Read the model definition and answer for the solid it produces. Units are mm, in the model's axes. A direction names the side the tool comes from. Coordinates: 2 decimals unless noted, no trailing zeros. Loops run counter-clockwise (first coordinate to the right, second up) from the corner with the lowest first, then second, coordinate; pieces in that order, holes last. Notation, with made-up numbers: M 36,-28 L 69,-28 A18 cw 69,-19 Z; hole C 5.5,-19 d3. An arc over 180 degrees is marked long. One line per item, written item: value. Start each with the question number.
1. The part is cut by section B-B (z = 3.45). Write down the section's boundary in (x, y) (3 decimals), then the cut area to 3 significant figures.
2. The part is cut by section D-D (y = 17). Write down the section's boundary in (x, z) (3 decimals).
3. The part is cut by section C-C (x = 62). Write down the section's boundary in (y, z) (3 decimals).
4. For faces 1 (the face through (39, 50.8, 3)), 2 (the face through (72.12, 46.67, 3.51)), 3 (the face through (6.979, 25, 1)), determine the directions among +Z, -Z, +X, -X, +Y, -Y from which every point of the face is accessible in a straight line to the end or side of a thin tool.
5. Determine the mould class of faces 4 (the face through (76.2, 25, 3)), 5 (the face through (39, 47.625, 4)), 6 (the face through (1.91, 48.99, 2.5)) for opening direction X: +X half, -X half, draft (parallel to the pull), parting line (faces both ways), or undercut.
6. Consider probe 1 along Y at (x, z) = (68.5, 3.4) (3 decimals); probe 2 along X at (y, z) = (34, 2) (3 decimals); probe 3 along Z at (x, y) = (41, 23.5) (3 decimals). Determine where each line is inside the solid, lowest interval first.
7. Flat-ended cylindrical pins translate along their axes: pin 1 (1.4 mm diameter, centred on x = 5, z = 1, fed in from +Y); pin 2 (0.6 mm diameter, centred on x = 5, z = 1, fed in from -Y). Find the tip coordinate at first contact, or state that the pin passes through.
8. The part is cut by section A-A (y = 24.5). Write down the section's boundary in (x, z) (3 decimals), then the cut area to 3 significant figures.
```python
from build123d import *

# Parameters (mm, degrees)
F1_DEPTH = 5.08
F3_DEPTH = 3.175
F5_DEPTH = 25.4


with BuildPart() as f1:
    # F0 (on Top) → F1 (new body)
    with BuildSketch(Plane.XY):
        with BuildLine():
            ThreePointArc((0, 6.35), (1.859872, 1.859872), (6.35, 0))
            Line((6.35, 0), (69.85, 0))
            ThreePointArc((69.85, 0), (74.340128, 1.859872), (76.2, 6.35))
            Line((76.2, 6.35), (76.2, 44.45))
            ThreePointArc((76.2, 44.45), (74.340128, 48.940128), (69.85, 50.8))
            Line((69.85, 50.8), (6.35, 50.8))
            ThreePointArc((6.35, 50.8), (1.859872, 48.940128), (0, 44.45))
            Line((0, 44.45), (0, 6.35))
        make_face()
    extrude(amount=F1_DEPTH)

    # F2 (on face) → F3 (cut)
    with BuildSketch(Plane.XY.offset(5.08)):
        with BuildLine():
            Line((69.85, 47.625), (6.35, 47.625))
            ThreePointArc((6.35, 47.625), (4.104936, 46.695064), (3.175, 44.45))
            Line((3.175, 44.45), (3.175, 6.35))
            ThreePointArc((3.175, 6.35), (4.104936, 4.104936), (6.35, 3.175))
            Line((6.35, 3.175), (69.85, 3.175))
            ThreePointArc((69.85, 3.175), (72.095064, 4.104936), (73.025, 6.35))
            Line((73.025, 6.35), (73.025, 44.45))
            ThreePointArc((73.025, 44.45), (72.095064, 46.695064), (69.85, 47.625))
        make_face()
    extrude(amount=-F3_DEPTH, mode=Mode.SUBTRACT)

    # F4 (on Top) → F5 (cut)
    with BuildSketch(Plane.XY):
        with BuildLine():
            Line((5.708611, 28.575), (4.445, 28.575))
            ThreePointArc((4.445, 28.575), (3.546974, 28.203026), (3.175, 27.305))
            Line((3.175, 27.305), (3.175, 23.495))
            ThreePointArc((3.175, 23.495), (3.546974, 22.596974), (4.445, 22.225))
            Line((4.445, 22.225), (5.708611, 22.225))
            ThreePointArc((5.708611, 22.225), (6.606637, 22.596974), (6.978611, 23.495))
            Line((6.978611, 23.495), (6.978611, 27.305))
            ThreePointArc((6.978611, 27.305), (6.606637, 28.203026), (5.708611, 28.575))
        make_face()
    extrude(amount=F5_DEPTH, mode=Mode.SUBTRACT)


solid = f1.part
```
Answer block:
1. outline: M 0,6.35 A6.35 ccw 6.35,0 L 69.85,0 A6.35 ccw 76.2,6.35 L 76.2,44.45 A6.35 ccw 69.85,50.8 L 6.35,50.8 A6.35 ccw 0,44.45 Z; hole M 3.175,6.35 A3.175 ccw 6.35,3.175 L 69.85,3.175 A3.175 ccw 73.025,6.35 L 73.025,44.45 A3.175 ccw 69.85,47.625 L 6.35,47.625 A3.175 ccw 3.175,44.45 Z
1. area: 740 mm2
2. outline: M 0,0 L 76.2,0 L 76.2,5.08 L 73.025,5.08 L 73.025,1.905 L 3.175,1.905 L 3.175,5.08 L 0,5.08 Z
3. outline: M 0,0 L 50.8,0 L 50.8,5.08 L 47.625,5.08 L 47.625,1.905 L 3.175,1.905 L 3.175,5.08 L 0,5.08 Z
4. face 1: +Z, -Z, +X, -X, +Y
4. face 2: +Z
4. face 3: +Z, -Z
5. face 4: +X half
5. face 5: undercut
5. face 6: -X half
6. probe 1: y = 0 to 3.175, 47.625 to 50.8
6. probe 2: x = 0 to 3.175, 73.025 to 76.2
6. probe 3: z = 0 to 1.905
7. pin 1: stops at y = 50.77
7. pin 2: stops at y = 0.09
8. outline: M 0,0 L 3.175,0 L 3.175,5.08 L 0,5.08 Z; M 6.979,0 L 76.2,0 L 76.2,5.08 L 73.025,5.08 L 73.025,1.905 L 6.979,1.905 Z
8. area: 158 mm2
